The model under review builds one solid part; all positions refer to its coordinate system, in mm. Face numbers are marked on the shaded views. A direction names the side the tool comes from. Give positions to 0.01 mm unless a question says otherwise; leave off trailing zeros. Write each loop counter-clockwise with the first axis right and the second up, starting at its lowest first coordinate (ties: lowest second). Pieces come first, ordered by that corner, then holes. Notation, with made-up numbers: (19, 41) -> (31, 41) arc R34 ccw to (31, 76) -> close; hole circle Ø6 at (84.5, 35). An arc over 180 degrees is marked (long way). Use CSV: the item, a comma, the result in double quotes.
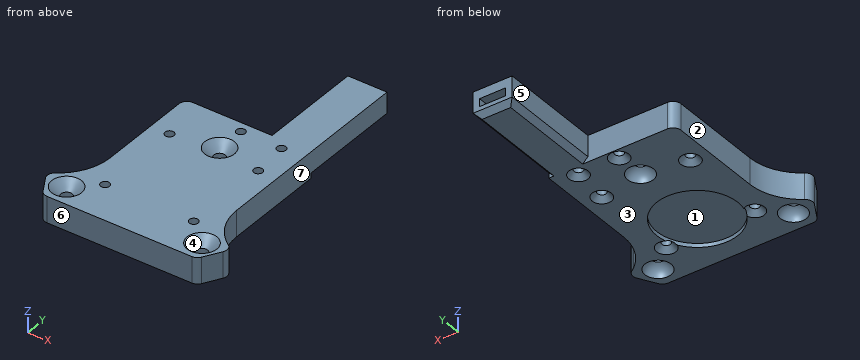
```python
from build123d import *

# Parameters (mm, degrees)
SKETCH2_R                                       = 7.5
BOSS_EXTRUDE1_DEPTH                             = 10
CSK_FOR_M4_FLAT_HEAD_MACHINE_SCREW1_D           = 4.3
CSK_FOR_M4_FLAT_HEAD_MACHINE_SCREW1_CSINK_D     = 11.4
CSK_FOR_M4_FLAT_HEAD_MACHINE_SCREW1_CSINK_ANGLE = 90
FILLET1_R                                       = 20
CIRPATTERN2_COUNT                               = 3
FILLET2_R                                       = 3
SKETCH47_R                                      = 1.7
CUT_EXTRUDE1_DEPTH                              = 58.559983963
SKETCH49_W                                      = 15
SKETCH49_H                                      = 10
SKETCH49_W_2                                    = 10
SKETCH49_H_2                                    = 3
BOSS_EXTRUDE2_DEPTH                             = 40
CHAMFER1_SIZE                                   = 2
BOSS_EXTRUDE3_REACH                             = 78.74
SKETCH51_W                                      = 3
SKETCH51_H                                      = 10
BOSS_EXTRUDE4_DEPTH                             = 10
SKETCH48_R                                      = 1.7
CUT_EXTRUDE2_DEPTH                              = 93.266742447
CHAMFER4_SIZE                                   = 2
CHAMFER3_SIZE                                   = 2
SKETCH53_R                                      = 15.5
CUT_EXTRUDE3_DEPTH                              = 1.5
SKETCH54_R                                      = 7.5
BOSS_EXTRUDE5_DEPTH                             = 8.5
CUT_EXTRUDE4_DEPTH                              = 93.266742447


with BuildPart() as part:
    # Sketch2 → Boss-Extrude1 (new body)
    with BuildSketch(Plane.XY):
        Polygon((-24.25, 45), (24.25, 45), (24.25, -5.917840259), (35.54293994, -12.437822174), (29.54293994, -22.830127019), (-29.54293994, -22.830127019), (-35.54293994, -12.437822174), (-24.25, -5.917840259), align=None)
        Circle(SKETCH2_R, mode=Mode.SUBTRACT)
    extrude(amount=BOSS_EXTRUDE1_DEPTH)

    # CSK for M4 Flat Head Machine Screw1 (through all)
    with Locations(Plane.XY.offset(10)):
        with Locations((-25.980762114, -15), (0, 30), (25.980762114, -15)):
            CounterSinkHole(CSK_FOR_M4_FLAT_HEAD_MACHINE_SCREW1_D / 2, CSK_FOR_M4_FLAT_HEAD_MACHINE_SCREW1_CSINK_D / 2, counter_sink_angle=CSK_FOR_M4_FLAT_HEAD_MACHINE_SCREW1_CSINK_ANGLE)

    # Fillet1
    fillet1_edges = [part.edges().sort_by_distance(p)[0] for p in [
        (24.25, -5.917840259, 5),
        (-24.25, -5.917840259, 5),
    ]]
    fillet(fillet1_edges, radius=FILLET1_R)

    # Sketch46 → tool ball cutout (revolve, cut)
    with BuildSketch(Plane(origin=(0, 30, 0), x_dir=(1, 0, 0), z_dir=(0, 1, 0))):
        with BuildLine():
            Line((0, 5.3), (0, -4.7))
            ThreePointArc((0, -4.7), (-5, 0.3), (0, 5.3))
        make_face()
    tool_ball_cutout = revolve(axis=Axis((0, 30, 0), (0, 0, -1)), mode=Mode.SUBTRACT)

    # CirPattern2: tool ball cutout ×3 about axis
    cirpattern2_axis = Axis((0, 0, 0), (0, 0, 1))
    for i in range(1, CIRPATTERN2_COUNT):
        add(tool_ball_cutout.rotate(cirpattern2_axis, i * 360 / CIRPATTERN2_COUNT), mode=Mode.SUBTRACT)

    # Fillet2
    fillet2_edges = [part.edges().sort_by_distance(p)[0] for p in [
        (24.25, 45, 5),
        (-24.25, 45, 5),
        (-29.54293994, -22.830127019, 5),
        (-35.54293994, -12.437822174, 5),
        (29.54293994, -22.830127019, 5),
        (35.54293994, -12.437822174, 5),
    ]]
    fillet(fillet2_edges, radius=FILLET2_R)

    # Sketch47 → Cut-Extrude1 (cut, through all)
    with BuildSketch(Plane(origin=(0, 0, 0), x_dir=(-1, 0, 0), z_dir=(0, 0, -1))):
        with Locations((-17, 27)):
            Circle(SKETCH47_R)
        with Locations((17, 27)):
            Circle(SKETCH47_R)
        with Locations((17, -7)):
            Circle(SKETCH47_R)
        with Locations((-17, -7)):
            Circle(SKETCH47_R)
    extrude(amount=-CUT_EXTRUDE1_DEPTH, mode=Mode.SUBTRACT)

    # Sketch49 → Boss-Extrude2 (add)
    with BuildSketch(Plane(origin=(0, 45, 0), x_dir=(1, 0, 0), z_dir=(0, 1, 0))):
        with Locations((16.75, -5)):
            Rectangle(SKETCH49_W, SKETCH49_H)
        with Locations((16.75, -5)):
            Rectangle(SKETCH49_W_2, SKETCH49_H_2, mode=Mode.SUBTRACT)
    extrude(amount=BOSS_EXTRUDE2_DEPTH)

    # Chamfer1
    chamfer1_edges = [part.edges().sort_by_distance(p)[0] for p in [
        (18.7, -7, 0),
        (-15.3, -7, 0),
        (-15.3, 27, 0),
        (18.7, 27, 0),
    ]]
    chamfer(chamfer1_edges, length=CHAMFER1_SIZE)

    # Sketch51 → Boss-Extrude3 (add, up to next)
    with BuildSketch(Plane.XZ.offset(-45), mode=Mode.PRIVATE) as boss_extrude3_sk1:
        with Locations((22.75, 5)):
            Rectangle(SKETCH51_W, SKETCH51_H)
    boss_extrude3_tool1 = extrude(boss_extrude3_sk1.sketch, amount=BOSS_EXTRUDE3_REACH, mode=Mode.PRIVATE) - part.part
    add(boss_extrude3_tool1.solids().sort_by_distance((22.75, 45, 5))[0])

    # Sketch52 → Boss-Extrude4 (add)
    with BuildSketch(Plane.XY.offset(10)):
        with BuildLine():
            Line((24.25, 45), (31.75, 45))
            Line((31.75, 45), (31.75, -9.983329871))
            ThreePointArc((31.75, -9.983329871), (26.222243623, -3.031088913), (24.25, 5.629165125))
            Line((24.25, 5.629165125), (24.25, 45))
        make_face()
    extrude(amount=-BOSS_EXTRUDE4_DEPTH)

    # Sketch48 → Cut-Extrude2 (cut, through all)
    with BuildSketch(Plane.XY.offset(10)):
        with Locations((0.150338606, 41)):
            Circle(SKETCH48_R)
        with Locations((15.750338606, 41)):
            Circle(SKETCH48_R)
    extrude(amount=-CUT_EXTRUDE2_DEPTH, mode=Mode.SUBTRACT)

    # Chamfer4
    chamfer4_edges = [part.edges().sort_by_distance(p)[0] for p in [
        (-1.549661394, 41, 0),
        (14.050338606, 41, 0),
    ]]
    chamfer(chamfer4_edges, length=CHAMFER4_SIZE)

    # Chamfer3
    chamfer3_edges = [part.edges().sort_by_distance(p)[0] for p in [
        (16.75, 85, 0),
        (9.25, 65, 0),
        (24.25, 65, 0),
    ]]
    chamfer(chamfer3_edges, length=CHAMFER3_SIZE)

    # Sketch53 → Cut-Extrude3 (cut)
    with BuildSketch(Plane(origin=(0, 0, 0), x_dir=(-1, 0, 0), z_dir=(0, 0, -1))):
        Circle(SKETCH53_R)
    extrude(amount=-CUT_EXTRUDE3_DEPTH, mode=Mode.SUBTRACT)

    # Sketch54 → Boss-Extrude5 (add)
    with BuildSketch(Plane(origin=(0, 0, 1.5), x_dir=(-1, 0, 0), z_dir=(0, 0, -1))):
        Circle(SKETCH54_R)
    extrude(amount=-BOSS_EXTRUDE5_DEPTH)

    # Sketch55 → Cut-Extrude4 (cut, through all)
    with BuildSketch(Plane(origin=(0, 0, 0), x_dir=(-1, 0, 0), z_dir=(0, 0, -1))):
        with BuildLine():
            Line((-24.25, 45), (-24.25, 5.629165125))
            ThreePointArc((-24.25, 5.629165125), (-26.222243623, -3.031088913), (-31.75, -9.983329871))
            Line((-31.75, -9.983329871), (-31.75, 45))
            Line((-31.75, 45), (-24.25, 45))
        make_face()
    extrude(amount=-CUT_EXTRUDE4_DEPTH, mode=Mode.SUBTRACT)


solid = part.part
```
Q1. Consider section A-A (x = -17). Write out the cut boundary in (y, z), then the cut area to 3 significant figures.
Derived:
outline,"(-22.83, 0) -> (-10.7, 0) -> (-8.7, 2) -> (-8.7, 10) -> (-22.83, 10) -> close; (-5.3, 2) -> (-3.3, 0) -> (23.3, 0) -> (25.3, 2) -> (25.3, 10) -> (-5.3, 10) -> close; (28.7, 2) -> (30.7, 0) -> (45, 0) -> (45, 10) -> (28.7, 10) -> close"
area,"602 mm2"
Q2. Machinability: for the marked faces 5, 6 and 7, which of the approach directions +Z, -Z, +X, -X, +Y, -Y give a long, thin tool a straight path to every point of the face, cutting with its end or side? Answer none if there is none.
Derived:
face 5,"+Z, -Z, -X, +Y"
face 6,"+Z, -Z, +X, -X, -Y"
face 7,"+Z, -Z, +X, +Y"
Q3. Consider section B-B (y = 53.5). Write out the cut boundary in (x, z), then the cut area to 3 significant figures.
Derived:
outline,"(9.25, 2) -> (11.25, 0) -> (22.25, 0) -> (24.25, 2) -> (24.25, 10) -> (9.25, 10) -> close; hole (11.75, 3.5) -> (21.75, 3.5) -> (21.75, 6.5) -> (11.75, 6.5) -> close"
area,"116 mm2"
Q4. The part is to be moulded in two halves that separate along X. For the marked faces 1, 2, 3 and 4, say which applies: pulls with the +X half, pulls with the -X half, needs draft (parallel to the pull), parting line crosses it, or undercut.
Derived:
face 1,"undercut"
face 2,"pulls with the -X half"
face 3,"needs draft"
face 4,"undercut"
Q5. Consider section C-C (x = 0). State how many separate pieces and enclosed holes the cut face has, then the cut area to 3 significant figures.
Derived:
separate pieces,"3"
enclosed holes,"0"
area,"522 mm2"
Q6. To check wall thickness, follow probe 1 along X at (y, z) = (-15, 5.2); probe 2 along X at (y, z) = (30, 5.2); probe 3 along Y at (x, z) = (16, 2.25). State the ranges of each line that lie inside material, in increasing order.
Derived:
probe 1,"x = -34.06 to -28.13, -23.83 to 23.83, 28.13 to 34.06"
probe 2,"x = -24.25 to -2.15, 2.15 to 24.25"
probe 3,"y = -22.83 to -8.37, -5.63 to 25.63, 28.37 to 39.32, 42.68 to 85"
Q7. Insertion check: pin 1 (3 mm diameter, centred on x = -17, y = 27, fed in from +Z); pin 2 (2 mm diameter, centred on x = -9.5, z = 1, fed in from +Y); pin 3 (1.5 mm diameter, centred on y = 65.5, z = 5.5, fed in from +X); pin 4 (5.5 mm diameter, centred on x = 0, y = 30, fed in from +Z). Each pin has a flat end and moves straight along its axis. Give the tip position at first contact, or say it passes through.
Derived:
pin 1,"passes through"
pin 2,"stops at y = 45"
pin 3,"stops at x = 24.25"
pin 4,"stops at z = 7.05"
